```python
from build123d import *

# Parameters (mm, degrees)
SKETCH1_R          = 1.5
EXTRUDE1_DEPTH     = 3
CUT_EXTRUDE1_START = -10
SKETCH2_R          = 1.5
CUT_EXTRUDE1_DEPTH = 10


with BuildPart() as part:
    # Sketch1 → Extrude1 (new body)
    with BuildSketch(Plane.XY):
        with BuildLine():
            Line((0, -5), (16, -5))
            ThreePointArc((16, -5), (21, 0), (16, 5))
            Line((16, 5), (0, 5))
            ThreePointArc((0, 5), (-5, 0), (0, -5))
        make_face()
        with Locations((16, 0)):
            Circle(SKETCH1_R, mode=Mode.SUBTRACT)
        Circle(SKETCH1_R, mode=Mode.SUBTRACT)
    extrude(amount=EXTRUDE1_DEPTH)

    # Sketch2 → Cut-Extrude1 (cut)
    with BuildSketch(Plane.XY.offset(3).offset(CUT_EXTRUDE1_START)):
        with Locations((16, 0)):
            Circle(SKETCH2_R)
        Polygon((0, 2.886751346), (-2.5, 1.443375673), (-2.5, -1.443375673), (0, -2.886751346), (2.5, -1.443375673), (2.5, 1.443375673), align=None)
        with BuildLine():
            Line((4.582575695, -2), (11.417424305, -2))
            ThreePointArc((11.417424305, -2), (11, 0), (11.417424305, 2))
            Line((11.417424305, 2), (4.582575695, 2))
            ThreePointArc((4.582575695, 2), (5, 0), (4.582575695, -2))
        make_face()
    extrude(amount=CUT_EXTRUDE1_DEPTH, mode=Mode.SUBTRACT)


solid = part.part
```
CAD build for the part. Positions are in the model's coordinates, mm. A direction names the side the tool comes from. Round coordinates to 2 decimals unless told otherwise and drop trailing zeros. Order: outer loops, then holes, each group sorted by start corner. A loop starts at its lowest first (then second) coordinate and runs counter-clockwise, first axis right, second up.
Q1. Slice it at A-A (x = 8.25). Write the cut outline in (y, z), and give its area (3 significant figures).
Q2. Drop flat-ended pins along their axis: pin 1 (1.5 mm diameter, centred on x = -0.5, z = 2.5, fed in from -Y); pin 2 (3 mm diameter, centred on x = 0.5, y = -0.5, fed in from +Z). Give the stop position or say it passes through.
Q3. Which spindle directions (+Z, -Z, +X, -X, +Y, -Y) get a long thin tool onto all of the face, cutting with end or side? Do faces 4 (the flat face through (-2.5, 0, 1)), 5 (the flat face through (8, -5, 1)). Say none if no direction does.
Q4. Slice it at D-D (x = 1). Write the cut outline in (y, z).
Q5. Slice it at B-B (y = 0). Write the cut outline in (x, z), and give its area (3 significant figures).
Q6. Two-plate mould, pull along X, no slides. Class faces 1 (the cylindrical face through (11, 0, 1)), 2 (the cylindrical face through (21, 0, 1)), 3 (the flat face through (8, 5, 1)): pulls with the +X half, pulls with the -X half, needs draft (parallel to the pull), parting line crosses it, or undercut.
Q7. Wall check: L1, parallel to Y at x = 16, z = 1.2; L2, parallel to Y at x = 6.25, z = 2.75; L3, parallel to X at y = 0.75, z = 1.25. Give the ranges that are in metal, low to high.
Q8. Slice it at C-C (z = 1.2). Write the cut outline in (x, y), and give its area (3 significant figures).
Results below:
1. outline: (-5, 0) - (-2, 0) - (-2, 3) - (-5, 3) - close; (2, 0) - (5, 0) - (5, 3) - (2, 3) - close
1. area: 18.0 mm2
2. pin 1: stops at y = -5
2. pin 2: passes through
3. face 4: +Z, -Z
3. face 5: +Z, -Z, +X, -X, -Y
4. outline: (-5, 0) - (-2.31, 0) - (-2.31, 3) - (-5, 3) - close; (2.31, 0) - (5, 0) - (5, 3) - (2.31, 3) - close
5. outline: (-5, 0) - (-2.5, 0) - (-2.5, 3) - (-5, 3) - close; (2.5, 0) - (5, 0) - (5, 3) - (2.5, 3) - close; (11, 0) - (14.5, 0) - (14.5, 3) - (11, 3) - close; (17.5, 0) - (21, 0) - (21, 3) - (17.5, 3) - close
5. area: 36.0 mm2
6. face 1: undercut
6. face 2: pulls with the +X half
6. face 3: needs draft
7. L1: y = -5 to -1.5, 1.5 to 5
7. L2: y = -5 to -2, 2 to 5
7. L3: x = -4.94 to -2.5, 2.5 to 4.94, 11.06 to 14.7, 17.3 to 20.94
8. outline: (0, -5) - (16, -5) arc R5 ccw to (16, 5) - (0, 5) arc R5 ccw to start; hole (-2.5, -1.44) - (0, -2.89) - (2.5, -1.44) - (2.5, 1.44) - (0, 2.89) - (-2.5, 1.44) - close; hole (4.58, -2) - (11.42, -2) arc R5 cw to (11.42, 2) - (4.58, 2) arc R5 cw to start; hole circle Ø3 at (16, 0)
8. area: 185 mm2
